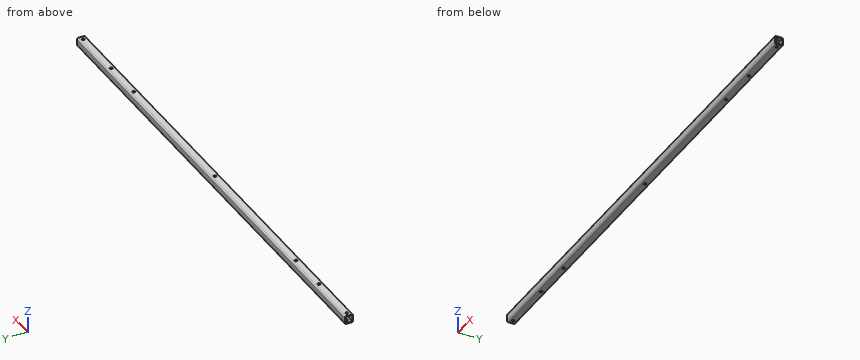
from build123d import *

# Parameters (mm, degrees)
F0_R     = 3.25
F1_DEPTH = 20
F2_W     = 16
F2_H     = 16
F3_DEPTH = 1220
F4_R     = 3


with BuildPart() as f1:
    # F0 (on Top) → F1 (new body)
    with BuildSketch(Plane.XY):
        Polygon((549.784225, -111.698022), (-658.215775, -111.698022), (-658.215775, -131.698022), (-49.215775, -131.698022), (319.784225, -131.698022), (422.784225, -131.698022), (559.784225, -131.698022), (559.784225, -121.698022), (559.784225, -111.698022), align=None)
        with Locations((-521.215775, -121.698022)):
            Circle(F0_R, mode=Mode.SUBTRACT)
        with Locations((-418.215775, -121.698022)):
            Circle(F0_R, mode=Mode.SUBTRACT)
        with Locations((-49.215775, -121.698022)):
            Circle(F0_R, mode=Mode.SUBTRACT)
        with Locations((319.784225, -121.698022)):
            Circle(F0_R, mode=Mode.SUBTRACT)
        with Locations((422.784225, -121.698022)):
            Circle(F0_R, mode=Mode.SUBTRACT)
        with Locations((-648.215775, -121.698022)):
            Circle(F0_R, mode=Mode.SUBTRACT)
        with Locations((549.784225, -121.698022)):
            Circle(F0_R, mode=Mode.SUBTRACT)
    extrude(amount=F1_DEPTH)

    # F2 (on face) → F3 (cut)
    with BuildSketch(Plane(origin=(-658.215775, 0, 0), x_dir=(0, -1, 0), z_dir=(-1, 0, 0))):
        with Locations((121.698022, 10)):
            Rectangle(F2_W, F2_H)
    extrude(amount=-F3_DEPTH, mode=Mode.SUBTRACT)

    # F4
    f4_edges = [f1.edges().sort_by_distance(p)[0] for p in [
        (-49.215775, -131.698022, 20),
        (-49.215775, -111.698022, 20),
        (-49.215775, -131.698022, 0),
        (-49.215775, -111.698022, 0),
    ]]
    fillet(f4_edges, radius=F4_R)


solid = f1.part
Can you work these out from the model? Positions are in its coordinate system, mm. Round coordinates to 2 decimals unless told otherwise and drop trailing zeros. Loops run counter-clockwise (first coordinate to the right, second up) from the corner with the lowest first, then second, coordinate; pieces in that order, holes last. Notation, with made-up numbers: (15, 2) - (57, 2) arc R29 cw to (57, 36) - close; hole circle Ø5 at (-0.75, 34.5). An arc over 180 degrees is marked (long way). Write item = value, one per line. Start each with the question number.
(1) For P1, Ø8.5, axis at x = 319.78, y = -121.7, coming from the +Z side; P2, Ø5, axis at x = -49.22, y = -121.7, coming from the -Z side, each with a flat end and sliding along its axis, tell me the tip position at first contact or that it passes through.
(2) If we section it at A-A (z = 11.75): Please give me the cut outline in (x, y), and give its area (3 significant figures).
(3) If we section it at B-B (x = 50): Please give me the cut outline in (y, z).
(4) If I drill on probe 1 along Y at (x, z) = (289.5, 2.75); probe 2 along Z at (x, y) = (-31, -118.5); probe 3 along Z at (x, y) = (-14.5, -129.5), over which ranges is the centre line in solid material (lowest first)? Write a range as [from, to].
Ans:
q1.P1 = 20
q1.P2 = through
q2.outline = (-658.22, -131.7) - (559.78, -131.7) - (559.78, -129.7) - (-658.22, -129.7) - close; (-658.22, -113.7) - (559.78, -113.7) - (559.78, -111.7) - (-658.22, -111.7) - close
q2.area = 4,870 mm²
q3.outline = (-131.7, 3) arc R3 ccw to (-128.7, 0) - (-114.7, 0) arc R3 ccw to (-111.7, 3) - (-111.7, 17) arc R3 ccw to (-114.7, 20) - (-128.7, 20) arc R3 ccw to (-131.7, 17) - close; hole (-129.7, 2) - (-113.7, 2) - (-113.7, 18) - (-129.7, 18) - close
q4.probe_1 = [-131.69, -129.7], [-113.7, -111.71]
q4.probe_2 = [0, 2], [18, 20]
q4.probe_3 = [0.11, 2], [18, 19.89]
